Verification items for the finished model (mm, model axes). A direction names the side the tool comes from. Coordinates: 2 decimals unless noted, no trailing zeros. Order: outer loops, then holes, each group sorted by start corner. A loop starts at its lowest first (then second) coordinate and runs counter-clockwise, first axis right, second up. Notation, with made-up numbers: M 8,15 L 52,15 A26 cw 52,51 Z; hole C 33.25,45 d1. An arc over 180 degrees is marked long. Return JSON: item names as keys, results as strings.
```python
from build123d import *

# Parameters (mm, degrees)
ESQUISSE1_W        = 2
ESQUISSE1_H        = 40
BOSS_EXTRU_1_DEPTH = 2.8


with BuildPart() as part:
    # Esquisse1 → Base-Révolution (revolve)
    with BuildSketch(Plane(origin=(0, 0, 0), x_dir=(1, 0, 0), z_dir=(0, 1, 0))):
        with Locations((1, -20)):
            Rectangle(ESQUISSE1_W, ESQUISSE1_H)
    revolve(axis=Axis((0, 0, 0), (0, 0, 1)))

    # Chanfrein1: read off the stored shape, not the designer's step
    # Chanfrein1 outline → Chanfrein1 (revolve, cut)
    with BuildSketch(Plane.XZ):
        Polygon((2, 40), (1.6, 40), (2, 39.6), align=None)
    revolve(axis=Axis((0, 0, 0), (0, 0, 1)), mode=Mode.SUBTRACT)

    # Esquisse6 → Boss.-Extru.1 (add)
    with BuildSketch(Plane.XY):
        Polygon((3.5, -2.020725942), (3.5, 2.020725942), (0, 4.041451884), (-3.5, 2.020725942), (-3.5, -2.020725942), (0, -4.041451884), align=None)
    extrude(amount=-BOSS_EXTRU_1_DEPTH)

    # Esquisse7 → Enlèvement de matière-Révolution1 (revolve, cut)
    with BuildSketch(Plane(origin=(0, 0, 0), x_dir=(1, 0, 0), z_dir=(0, 1, 0))):
        Polygon((-3.5, 2.8), (-8.349742261, 2.8), (-8.349742261, 0), align=None)
    revolve(axis=Axis((0, 0, -6.239446496), (0, 0, 1)), mode=Mode.SUBTRACT)


solid = part.part
```
Q1. Cross-section at A-A, the plane z = 14.5. Record the boundary of the cut face in (x, y), and give its area (3 significant figures).
Values:
{"outline": "C 0,0 d4", "area": "12.6 mm^2"}
Q2. Go/stop test with flat-tipped pins: pin 1 (4 mm diameter, centred on y = 0, z = 35, fed in from -X); pin 2 (1.5 mm diameter, centred on y = -2.5, z = 31.5, fed in from -X); pin 3 (1.5 mm diameter, centred on y = -1, z = 22.5, fed in from +X). Record where each tip stops, or that it passes through.
Values:
{"pin 1": "x = -2", "pin 2": "x = -0.97", "pin 3": "x = 1.98"}
Q3. Material ranges on line 1 along Z through (x, y) = (3, 1); line 2 along Y through (x, z) = (0, 27.5); line 3 along Y through (x, z) = (-0.5, 22), recorded low to high.
Values:
{"line 1": "-2.8 to 0", "line 2": "-2 to 2", "line 3": "-1.94 to 1.94"}
Q4. Tool access check on faces 1 (the face through (3.5, 0, -1)), 2 (the face through (0, -2, 20)). Record the directions out of +Z, -Z, +X, -X, +Y, -Y that give a thin tool (end or side, any length) a straight path to the whole face; none if there is none.
Values:
{"face 1": "+Z, -Z, +X, +Y, -Y", "face 2": "+Z"}
